from build123d import *

# Parameters (mm, degrees)
SKETCH1_R           = 152.4
BOSS_EXTRUDE1_DEPTH = 6.35
SKETCH2_R           = 4.1
CUT_EXTRUDE1_DEPTH  = 7.35
CIRPATTERN1_COUNT   = 3


with BuildPart() as part:
    # Sketch1 → Boss-Extrude1 (new body)
    with BuildSketch(Plane(origin=(0, 0, 0), x_dir=(1, 0, 0), z_dir=(0, 1, 0))):
        Circle(SKETCH1_R)
    extrude(amount=BOSS_EXTRUDE1_DEPTH)

    # Sketch2 → Cut-Extrude1 (cut, through all)
    with BuildSketch(Plane(origin=(0, 6.35, 0), x_dir=(1, 0, 0), z_dir=(0, 1, 0))):
        with Locations((0, 140)):
            Circle(SKETCH2_R)
    cut_extrude1 = extrude(amount=-CUT_EXTRUDE1_DEPTH, mode=Mode.SUBTRACT)

    # CirPattern1: Cut-Extrude1 ×3 about axis
    cirpattern1_axis = Axis((0, 0, 0), (0, 1, 0))
    for i in range(1, CIRPATTERN1_COUNT):
        add(cut_extrude1.rotate(cirpattern1_axis, i * 360 / CIRPATTERN1_COUNT), mode=Mode.SUBTRACT)


solid = part.part
The listing builds one solid part. Answer for the finished solid, in the listing's coordinates (mm). Round coordinates to 2 decimals unless told otherwise and drop trailing zeros. Loops run counter-clockwise (first coordinate to the right, second up) from the corner with the lowest first, then second, coordinate; pieces in that order, holes last. Notation, with made-up numbers: M -33.75,-29.5 L -21.75,-29.5 A19 ccw -21.75,-17.5 Z; hole C -18.5,75 d5. An arc over 180 degrees is marked long. Return JSON: item names as keys, results as strings.
Q1. Find section A-A, the plane x = 0. Determine the outline of the cut face in (y, z).
Results list:
{"outline": "M 0,-152.4 L 6.35,-152.4 L 6.35,-144.1 L 0,-144.1 Z; M 0,-135.9 L 6.35,-135.9 L 6.35,152.4 L 0,152.4 Z"}
Q2. Find section C-C, the plane z = 70. Determine the outline of the cut face in (x, y).
Results list:
{"outline": "M -135.37,0 L -125.34,0 L -125.34,6.35 L -135.37,6.35 Z; M -117.14,0 L 117.14,0 L 117.14,6.35 L -117.14,6.35 Z; M 125.34,0 L 135.37,0 L 135.37,6.35 L 125.34,6.35 Z"}
Q3. Find the intervals of material crossed by line 1 along Z through (x, y) = (0, 3); line 2 along Z through (x, y) = (121, 3.75); line 3 along X through (y, z) = (3, -140), in increasing order. Write a range as from..to.
Results list:
{"line 1": "z = -152.4..-144.1, -135.9..152.4", "line 2": "z = -92.65..65.91, 74.09..92.65", "line 3": "x = -60.21..-4.1, 4.1..60.21"}
Q4. Find section D-D, the plane y = 5.25. Determine the outline of the cut face in (x, z), plus the area to 3 significant figures.
Results list:
{"outline": "C 0,0 d304.8; hole C -121.24,70 d8.2; hole C 0,-140 d8.2; hole C 121.24,70 d8.2", "area": "72,800 mm2"}
Q5. Each of these flat-tipped pins is pushed along its axis until it touches: pin 1 Ø1 at (y, z) = (1.5, 60) entering from +X; pin 2 Ø1 at (x, y) = (34, 4.5) entering from +Z; pin 3 Ø1 at (x, y) = (3, 5) entering from -Z. Where does it stop, or does it pass through?
Results list:
{"pin 1": "stops at x = 140.31", "pin 2": "stops at z = 148.67", "pin 3": "stops at z = -152.38"}
Q6. The mould has two halves that part along Z. Classify faces 1 (the face through (-120.94, 3.13, 92.73)), 2 (the face through (-2, 0, -2)), 3 (the face through (-0.534, 3.219, -144.065)): released by +Z, released by -Z, zero draft, split by the parting line, or undercut.
Results list:
{"face 1": "split by the parting line", "face 2": "zero draft", "face 3": "undercut"}
Q7. Find section B-B, the plane z = -140. Determine the outline of the cut face in (x, y).
Results list:
{"outline": "M -60.21,0 L -4.1,0 L -4.1,6.35 L -60.21,6.35 Z; M 4.1,0 L 60.21,0 L 60.21,6.35 L 4.1,6.35 Z"}
